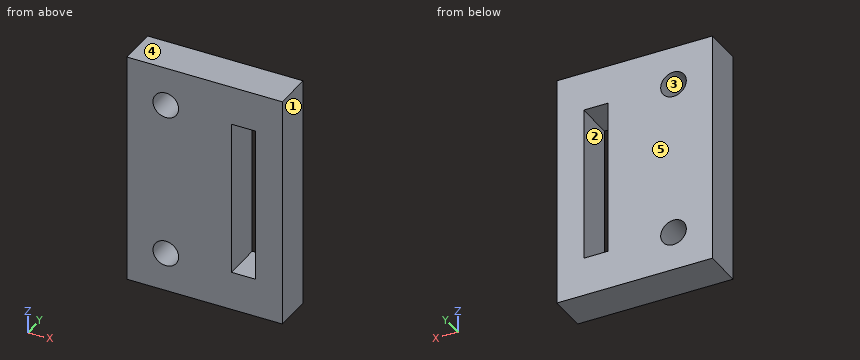
from build123d import *

# Parameters (mm, degrees)
SKETCH1_W           = 10
SKETCH1_H           = 15
SKETCH1_R           = 1.65
BOSS_EXTRUDE1_DEPTH = 5


with BuildPart() as part:
    # Sketch1 → Boss-Extrude1 (new body)
    # profile 1 of 4: a face of its own
    with BuildSketch(Plane(origin=(0, 0, 0), x_dir=(1, 0, 0), z_dir=(0, 1, 0))):
        with Locations((5, 22.5)):
            Rectangle(SKETCH1_W, SKETCH1_H)
        with Locations(Location((5, 25, 0), (0, 0, 270))):
            Circle(SKETCH1_R, mode=Mode.SUBTRACT)
    # profile 2 of 4: a face of its own
    with BuildSketch(Plane(origin=(0, 0, 0), x_dir=(1, 0, 0), z_dir=(0, 1, 0))):
        Polygon((10, 30), (10, 15), (13.45, 15), (13.45, 25), (16.55, 25), (16.55, 15), (20, 15), (20, 30), align=None)
    # profile 3 of 4: a face of its own
    with BuildSketch(Plane(origin=(0, 0, 0), x_dir=(1, 0, 0), z_dir=(0, 1, 0))):
        Polygon((13.45, 15), (10, 15), (10, 0), (20, 0), (20, 15), (16.55, 15), (16.55, 5), (13.45, 5), align=None)
    # profile 4 of 4: a face of its own
    with BuildSketch(Plane(origin=(0, 0, 0), x_dir=(1, 0, 0), z_dir=(0, 1, 0))):
        with Locations((5, 7.5)):
            Rectangle(SKETCH1_W, SKETCH1_H)
        with Locations(Location((5, 5, 0), (0, 0, 270))):
            Circle(SKETCH1_R, mode=Mode.SUBTRACT)
    extrude(amount=BOSS_EXTRUDE1_DEPTH)


solid = part.part
Input: part model. Units: mm. Frame: model coordinates. Face numbers are marked on the shaded views. A direction names the side the tool comes from. Give positions to 0.01 mm unless a question says otherwise; leave off trailing zeros. Write each loop counter-clockwise with the first axis right and the second up, starting at its lowest first coordinate (ties: lowest second). Pieces come first, ordered by that corner, then holes. Notation, with made-up numbers: (26.25, 13.5) -> (63.25, 13.5) arc R29 ccw to (63.25, 37.5) -> close; hole circle Ø4 at (-24, 32). An arc over 180 degrees is marked (long way). Use one line per item in the form item = value. Start each with the question number.
1) Section query D-D on y = 3.45. Return the cut outline in (x, z).
2) Draft query along Z for the marked faces 3, 4 and 5. Return one class per face: pulls with the +Z half, pulls with the -Z half, needs draft (parallel to the pull), parting line crosses it, or undercut.
3) Section query A-A on x = 14.25. Return the cut outline in (y, z), then the cut area to 3 significant figures.
4) Section query C-C on x = 5. Return the cut outline in (y, z).
5) Ray query, probe 1 along X at (y, z) = (2.2, -8.25); probe 2 along Z at (x, y) = (4, 2.85); probe 3 along Z at (x, y) = (6.25, 4.75). Return the intervals inside material, ascending. Write a range as from..to.
6) Set-up query: the marked faces 1 and 2. Return all of +Z, -Z, +X, -X, +Y, -Y with unobstructed straight access to the full face (end or side cutting, diameter ignored); none if empty.
7) Section query B-B on z = -16.5. Return the cut outline in (x, y), then the cut area to 3 significant figures.
Outcome:
q1.outline = (0, -30) -> (20, -30) -> (20, 0) -> (0, 0) -> close; hole circle Ø3.3 at (5, -25); hole circle Ø3.3 at (5, -5); hole (13.45, -25) -> (16.55, -25) -> (16.55, -5) -> (13.45, -5) -> close
q2.face_3 = undercut
q2.face_4 = pulls with the +Z half
q2.face_5 = needs draft
q3.outline = (0, -30) -> (5, -30) -> (5, -25) -> (0, -25) -> close; (0, -5) -> (5, -5) -> (5, 0) -> (0, 0) -> close
q3.area = 50.0 mm^2
q4.outline = (0, -30) -> (5, -30) -> (5, -26.65) -> (0, -26.65) -> close; (0, -23.35) -> (5, -23.35) -> (5, -6.65) -> (0, -6.65) -> close; (0, -3.35) -> (5, -3.35) -> (5, 0) -> (0, 0) -> close
q5.probe_1 = 0..13.45, 16.55..20
q5.probe_2 = -30..-26.31, -23.69..-6.31, -3.69..0
q5.probe_3 = -30..-26.08, -23.92..-6.08, -3.92..0
q6.face_1 = +Z, -Z, +X, +Y, -Y
q6.face_2 = +Y, -Y
q7.outline = (0, 0) -> (13.45, 0) -> (13.45, 5) -> (0, 5) -> close; (16.55, 0) -> (20, 0) -> (20, 5) -> (16.55, 5) -> close
q7.area = 84.5 mm^2
